from build123d import *

# Parameters (mm, degrees)
SKETCH1_R                = 21
SKETCH1_R_2              = 3.5
BOSS_EXTRUDE2_DEPTH      = 2
SKETCH1_4_R              = 22.5
SKETCH1_4_R_2            = 21
BOSS_EXTRUDE3_DEPTH      = 20
BOSS_EXTRUDE4_DEPTH      = 20
FILLET1_R                = 0.5
CIRPATTERN1_COUNT        = 16
FILLET1_OF_CIRPATTERN1_R = 0.5
SKETCH1_6_R              = 3.5
BOSS_EXTRUDE5_DEPTH      = 10
DRAFT1_ANGLE             = -1


with BuildPart() as part:
    # Sketch1 → Boss-Extrude2 (new body)
    with BuildSketch(Plane.XY):
        Circle(SKETCH1_R)
        Circle(SKETCH1_R_2, mode=Mode.SUBTRACT)
    extrude(amount=BOSS_EXTRUDE2_DEPTH)

    # Sketch1<4> → Boss-Extrude3 (add)
    with BuildSketch(Plane.XY):
        Circle(SKETCH1_4_R)
        Circle(SKETCH1_4_R_2, mode=Mode.SUBTRACT)
    extrude(amount=BOSS_EXTRUDE3_DEPTH)

    # Sketch1<5> → Boss-Extrude4 (add)
    with BuildSketch(Plane.XY):
        with BuildLine():
            ThreePointArc((0.13161991, 24.999653522), (-0.719679971, 24.989639068), (-1.570145241, 24.950644158))
            Line((-1.570145241, 24.950644158), (-0.161901615, 22.499417501))
            ThreePointArc((-0.161901615, 22.499417501), (0.719815444, 22.488482957), (1.600426946, 22.443008568))
            Line((1.600426946, 22.443008568), (0.13161991, 24.999653522))
        make_face()
    boss_extrude4 = extrude(amount=BOSS_EXTRUDE4_DEPTH)

    # Fillet1
    fillet1_edges = [part.edges().sort_by_distance(p)[0] for p in [
        (-0.161901615, 22.499417501, 10),
        (1.600426946, 22.443008568, 10),
        (0.13161991, 24.999653522, 10),
        (-1.570145241, 24.950644158, 10),
    ]]
    fillet(fillet1_edges, radius=FILLET1_R)

    # CirPattern1: Boss-Extrude4 ×16 about axis
    cirpattern1_axis = Axis((0, 0, 0), (0, 0, 1))
    for i in range(1, CIRPATTERN1_COUNT):
        add(boss_extrude4.rotate(cirpattern1_axis, i * 360 / CIRPATTERN1_COUNT))

    # Fillet1 of CirPattern1
    fillet1_of_cirpattern1_edges = [part.edges().sort_by_distance(p)[0] for p in [
        (-8.759731904, 20.724794257, 10),
        (-7.109965853, 21.347093141, 10),
        (-9.445352276, 23.147036968, 10),
        (-10.998823198, 22.450520891, 10),
        (-16.023972417, 15.795008958, 10),
        (-14.737930803, 17.001276295, 10),
        (-17.584355201, 17.770493864, 10),
        (-18.753030027, 16.532509332, 10),
        (-20.848708388, 8.460576727, 10),
        (-20.122179387, 10.06716925, 10),
        (-23.046299449, 9.688554159, 10),
        (-23.652258031, 8.097573095, 10),
        (-22.499417501, -0.161901615, 10),
        (-22.443008568, 1.600426946, 10),
        (-24.999653522, 0.13161991, 10),
        (-24.950644158, -1.570145241, 10),
        (-20.724794257, -8.759731904, 10),
        (-21.347093141, -7.109965853, 10),
        (-23.147036968, -9.445352276, 10),
        (-22.450520891, -10.998823198, 10),
        (-15.795008958, -16.023972417, 10),
        (-17.001276295, -14.737930803, 10),
        (-17.770493864, -17.584355201, 10),
        (-16.532509332, -18.753030027, 10),
        (-8.460576727, -20.848708388, 10),
        (-10.06716925, -20.122179387, 10),
        (-9.688554159, -23.046299449, 10),
        (-8.097573095, -23.652258031, 10),
        (0.161901615, -22.499417501, 10),
        (-1.600426946, -22.443008568, 10),
        (-0.13161991, -24.999653522, 10),
        (1.570145241, -24.950644158, 10),
        (8.759731904, -20.724794257, 10),
        (7.109965853, -21.347093141, 10),
        (9.445352276, -23.147036968, 10),
        (10.998823198, -22.450520891, 10),
        (16.023972417, -15.795008958, 10),
        (14.737930803, -17.001276295, 10),
        (17.584355201, -17.770493864, 10),
        (18.753030027, -16.532509332, 10),
        (20.848708388, -8.460576727, 10),
        (20.122179387, -10.06716925, 10),
        (23.046299449, -9.688554159, 10),
        (23.652258031, -8.097573095, 10),
        (22.499417501, 0.161901615, 10),
        (22.443008568, -1.600426946, 10),
        (24.999653522, -0.13161991, 10),
        (24.950644158, 1.570145241, 10),
        (20.724794257, 8.759731904, 10),
        (21.347093141, 7.109965853, 10),
        (23.147036968, 9.445352276, 10),
        (22.450520891, 10.998823198, 10),
        (15.795008958, 16.023972417, 10),
        (17.001276295, 14.737930803, 10),
        (17.770493864, 17.584355201, 10),
        (16.532509332, 18.753030027, 10),
        (8.460576727, 20.848708388, 10),
        (10.06716925, 20.122179387, 10),
        (9.688554159, 23.046299449, 10),
        (8.097573095, 23.652258031, 10),
    ]]
    fillet(fillet1_of_cirpattern1_edges, radius=FILLET1_OF_CIRPATTERN1_R)

    # Sketch1<6> → Boss-Extrude5 (add)
    with BuildSketch(Plane.XY):
        Circle(SKETCH1_6_R)
        with BuildLine():
            Line((-1.118033989, 1), (1.118033989, 1))
            ThreePointArc((1.118033989, 1), (0, -1.5), (-1.118033989, 1))
        make_face(mode=Mode.SUBTRACT)
    extrude(amount=BOSS_EXTRUDE5_DEPTH)

    # Draft1
    draft1_faces = [part.faces().sort_by_distance(p)[0] for p in [
        (0, 1, 5),
        (0, -1.5, 5),
    ]]
    draft(draft1_faces, Plane.XY.offset(10), DRAFT1_ANGLE)


solid = part.part
Source: CAD feature listing. Evaluate the final solid. Frame: model axes, mm. A direction names the side the tool comes from. Give positions to 0.01 mm unless a question says otherwise; leave off trailing zeros. Loops run counter-clockwise (first coordinate to the right, second up) from the corner with the lowest first, then second, coordinate; pieces in that order, holes last. Notation, with made-up numbers: (35, -25) -> (89, -25) arc R10 ccw to (89, -8) -> close; hole circle Ø7 at (73, -16.75). An arc over 180 degrees is marked (long way). Use a Markdown table: item, result. Add a question column.
1) First-contact query: pin 1 (6 mm diameter, centred on x = -12, y = 2, fed in from +Z); pin 2 (3.5 mm diameter, centred on x = -1, y = 0.5, fed in from +Z); pin 3 (5 mm diameter, centred on y = -9, z = 11.5, fed in from -X). Flat tips, straight axial feed; report the tip coordinate or a pass-through.
2) Reachability of faces 1 (the face through (16.17, 17.41, 9.86)), 2 (the face through (3.233, -1.341, 5.944)), 3 (the face through (-17.378, -16.133, 9.86)) from +Z, -Z, +X, -X, +Y, -Y: full face, straight path, thin tool, end or side. Return the list, or none.
3) Pull-direction query (Y, two-part tool) for faces 4 (the face through (-15, 15, 20)), 5 (the face through (-22.268, 8.277, 9.86)), 6 (the face through (-16.17, -17.41, 9.86)); classes: +Y half, -Y half, draft (parallel to the pull), parting line (faces both ways), or undercut.
4) Section query A-A, the plane z = 5.75. Count the separate pieces of the cut face and the enclosed holes in it, then the cut area to 3 significant figures.
5) Line query: line 1 along Y through (x, z) = (0, 16.5); line 2 along X through (y, z) = (9.5, 14); line 3 along X through (y, z) = (-18, 11.5). Output: solid intervals per line, ascending. Write a range as [from, to].
6) Section query B-B, the plane y = 13.5. Return the cut outline in (x, z).
Numbers:
| question | item | result |
|---|---|---|
| 1 | pin 1 | stops at z = 2 |
| 1 | pin 2 | stops at z = 10 |
| 1 | pin 3 | stops at x = -23.07 |
| 2 | face 1 | +Z, -Z, +Y |
| 2 | face 2 | +Z |
| 2 | face 3 | +Z, -Z, -X |
| 3 | face 4 | draft |
| 3 | face 5 | undercut |
| 3 | face 6 | -Y half |
| 4 | separate pieces | 2 |
| 4 | enclosed holes | 2 |
| 4 | area | 306 mm2 |
| 5 | line 1 | y = [-24.97, -21], [21, 24.97] |
| 5 | line 2 | x = [-23.12, -18.73], [18.73, 20.4], [21.3, 23.07] |
| 5 | line 3 | x = [-17.35, -16.33], [-13.5, -10.82], [10.82, 13.5] |
| 6 | outline | (-18, 0) -> (18, 0) -> (18, 20) -> (16.09, 20) -> (16.09, 2) -> (-16.09, 2) -> (-16.09, 20) -> (-18, 20) -> close |
